Work out the finished part from the listing and answer in its coordinate system (mm). A direction names the side the tool comes from. Coordinates: 2 decimals unless noted, no trailing zeros. Order: outer loops, then holes, each group sorted by start corner. A loop starts at its lowest first (then second) coordinate and runs counter-clockwise, first axis right, second up. Notation, with made-up numbers: (70.5, 9) -> (107.5, 9) arc R15 ccw to (107.5, 34) -> close; hole circle Ø7 at (89.5, 30). An arc over 180 degrees is marked (long way). Answer as CSV lines item,"result". Start each with the question number.
Item 1: Section B-B (y = -9.5) is taken. Count the separate pieces of the cut face and the enclosed holes in it, then the cut area to 3 significant figures.
Item 2: Section C-C (x = -3.5) is taken. Write down the section's boundary in (y, z) (3 decimals), then the cut area to 3 significant figures.
Item 3: Which of the six approach directions +Z, -Z, +X, -X, +Y, -Y give full straight-line access (tool end or side, diameter ignored) to faces 5 (the face through (-56.882, 5.964, -0.089)), 6 (the face through (-1, 15.875, -4)), 7 (the face through (61.61, 7.814, -0.325))?
Item 4: For a pull along X with two mould halves and no side action, classify faces 1 (the face through (37.49, -12.12, -1.19)), 2 (the face through (-43.66, 12.01, -0.17)), 3 (the face through (-63.78, 12.82, -0.09)), 4 (the face through (-1, -15.875, -4)) as pulls with the +X half, pulls with the -X half, needs draft (parallel to the pull), parting line crosses it, or undercut.
Item 5: Each of these flat-tipped pins is pushed along its axis until it touches: pin 1 Ø5 at (x, z) = (-47.625, 0) entering from -Y; pin 2 Ø2.5 at (y, z) = (6.35, 0) entering from +X; pin 3 Ø5 at (y, z) = (12, 5) entering from -X. Where does it stop, or does it pass through?
Item 6: Section A-A (x = -48) is taken. Write down the section's boundary in (y, z) (3 decimals).
Item 7: Straight lines are drawn through the part: L1, parallel to Y at x = 22, z = -4.5 (3 decimals); L2, parallel to Z at x = 61.75, y = 0 (3 decimals); L3, parallel to X at y = 11.5, z = 1.25. For each, find the intervals that lie inside material, in ascending order.
```python
from build123d import *

# Parameters (mm, degrees)
SKETCH1_W               = 133.35
SKETCH1_H               = 31.75
SKETCH1_W_2             = 118.11
SKETCH1_H_2             = 16.51
BOSS_EXTRUDE1_DEPTH     = 6.35
FILLET2_R               = 7.62
CUT_EXTRUDE1_DEPTH      = 69.832359759
CUT_EXTRUDE1_DEPTH_BACK = 69.832359759
SKETCH2_R               = 3.175
F_3_8_16_TAPPED_HOLE1_D = 7.9375
SKETCH5_R               = 1.5
CUT_EXTRUDE2_DEPTH      = 69.832359888
FILLET3_R               = 10.16
FILLET4_R               = 10.16
FILLET5_R               = 10.16
FILLET6_R               = 10.16


with BuildPart() as part:
    # Sketch1 → Boss-Extrude1 (new, symmetric)
    with BuildSketch(Plane.XY):
        Rectangle(SKETCH1_W, SKETCH1_H)
        Rectangle(SKETCH1_W_2, SKETCH1_H_2, mode=Mode.SUBTRACT)
    extrude(amount=BOSS_EXTRUDE1_DEPTH, both=True)

    # Fillet2
    fillet2_edges = [part.edges().sort_by_distance(p)[0] for p in [
        (59.055, -8.255, 0),
        (59.055, 8.255, 0),
        (-59.055, 8.255, 0),
        (-59.055, -8.255, 0),
    ]]
    fillet(fillet2_edges, radius=FILLET2_R)

    # Sketch2 → Cut-Extrude1 (cut, two sides: drawn at the far end of the back side and taken through both)
    with BuildSketch(Plane(origin=(0, 0, 0), x_dir=(0, 0, -1), z_dir=(1, 0, 0)).offset(-CUT_EXTRUDE1_DEPTH_BACK)):
        Circle(SKETCH2_R)
    extrude(amount=CUT_EXTRUDE1_DEPTH + CUT_EXTRUDE1_DEPTH_BACK, mode=Mode.SUBTRACT)

    # 3/8-16 Tapped Hole1 (through all)
    with Locations(Plane(origin=(0, 15.875, 0), x_dir=(1, 0, 0), z_dir=(0, 1, 0))):
        with Locations((-47.625, 0), (-3.175, 0), (41.275, 0)):
            Hole(F_3_8_16_TAPPED_HOLE1_D / 2)

    # Sketch5 → Cut-Extrude2 (cut, through all)
    with BuildSketch(Plane(origin=(0, 0, 0), x_dir=(0, 0, -1), z_dir=(1, 0, 0))):
        with Locations(Location((0, -6.35, 0), (0, 0, 180))):
            Circle(SKETCH5_R)
        with Locations(Location((0, 6.35, 0), (0, 0, 180))):
            Circle(SKETCH5_R)
    extrude(amount=CUT_EXTRUDE2_DEPTH, mode=Mode.SUBTRACT)

    # Fillet3
    fillet3_edges = [part.edges().sort_by_distance(p)[0] for p in [
        (-66.675, 15.875, 0),
    ]]
    fillet(fillet3_edges, radius=FILLET3_R)

    # Fillet4
    fillet4_edges = [part.edges().sort_by_distance(p)[0] for p in [
        (-66.675, -15.875, 0),
    ]]
    fillet(fillet4_edges, radius=FILLET4_R)

    # Fillet5
    # the kernel refuses this fillet: 10.16 mm, written as the material it takes off along each edge
    with BuildSketch(Plane(origin=(66.675, -15.875, -31.75), x_dir=(-1, 0, 0), z_dir=(0, 0, 1))) as fillet5_piece_1:
        with BuildLine():
            CenterArc((FILLET5_R, -FILLET5_R), FILLET5_R, 90, 90)
            Line((0, -FILLET5_R), (0, 0))
            Line((0, 0), (FILLET5_R, 0))
        make_face()
    extrude(amount=63.5, mode=Mode.SUBTRACT)

    # Fillet6
    # the kernel refuses this fillet: 10.16 mm, written as the material it takes off along each edge
    with BuildSketch(Plane(origin=(66.675, 15.875, 31.75), x_dir=(0, -1, 0), z_dir=(0, 0, -1))) as fillet6_piece_1:
        with BuildLine():
            CenterArc((FILLET6_R, FILLET6_R), FILLET6_R, 180, 90)
            Line((0, FILLET6_R), (0, 0))
            Line((0, 0), (FILLET6_R, 0))
        make_face()
    extrude(amount=63.5, mode=Mode.SUBTRACT)


solid = part.part
```
Checked values:
1,separate pieces,"1"
1,enclosed holes,"3"
1,area,"1,530 mm^2"
2,outline,"(-15.875, -6.35) -> (-8.255, -6.35) -> (-8.255, -3.955) -> (-15.875, -3.955) -> close; (-15.875, 3.955) -> (-8.255, 3.955) -> (-8.255, 6.35) -> (-15.875, 6.35) -> close; (8.255, -6.35) -> (15.875, -6.35) -> (15.875, -3.955) -> (8.255, -3.955) -> close; (8.255, 3.955) -> (15.875, 3.955) -> (15.875, 6.35) -> (8.255, 6.35) -> close"
2,area,"73.0 mm^2"
3,face 5,"+Z, -Z"
3,face 6,"+Z, -Z, +X, -X, +Y"
3,face 7,"+X"
4,face 1,"undercut"
4,face 2,"undercut"
4,face 3,"pulls with the -X half"
4,face 4,"needs draft"
5,pin 1,"passes through"
5,pin 2,"stops at x = -54.53"
5,pin 3,"stops at x = -65.94"
6,outline,"(-15.875, -6.35) -> (-8.255, -6.35) -> (-8.255, -3.951) -> (-15.875, -3.951) -> close; (-15.875, 3.951) -> (-8.255, 3.951) -> (-8.255, 6.35) -> (-15.875, 6.35) -> close; (8.255, -6.35) -> (15.875, -6.35) -> (15.875, -3.951) -> (8.255, -3.951) -> close; (8.255, 3.951) -> (15.875, 3.951) -> (15.875, 6.35) -> (8.255, 6.35) -> close"
7,L1,"y = -15.875 to -8.255, 8.255 to 15.875"
7,L2,"z = -6.35 to -3.175, 3.175 to 6.35"
7,L3,"x = -64.87 to -51.39, -43.86 to -6.94, 0.59 to 37.51, 45.04 to 64.87"
